For this review, take the finished solid that the model builds, in its own axes (mm). Coordinates: 2 decimals unless noted, no trailing zeros. Order: outer loops, then holes, each group sorted by start corner. A loop starts at its lowest first (then second) coordinate and runs counter-clockwise, first axis right, second up. Notation, with made-up numbers: M 50.5,21.25 L 76.5,21.25 A21 ccw 76.5,29.25 Z; hole C -30,57.5 d10. An arc over 180 degrees is marked long. Use one line per item in the form item = value. Start each with the question number.
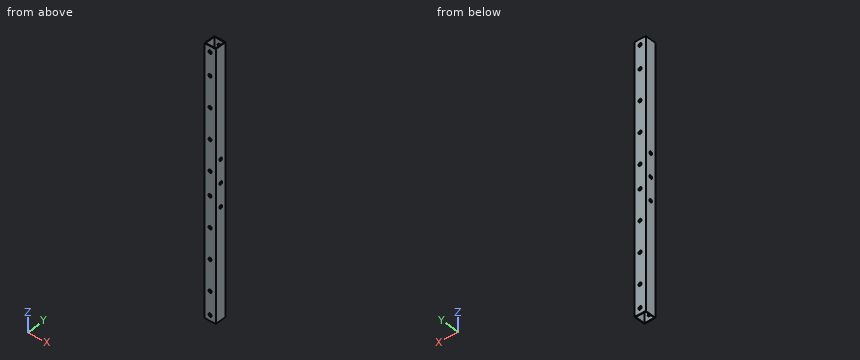
```python
from build123d import *

# Parameters (mm, degrees)
SKETCH_1_W          = 15
SKETCH_1_H          = 15
SKETCH_1_W_2        = 13
SKETCH_1_H_2        = 13
EXTRUDE_1_DEPTH     = 346
SKETCH_3_R          = 2.1
CUT_EXTRUDE_2_DEPTH = 55
SKETCH_4_R          = 2.1
CUT_EXTRUDE_3_DEPTH = 55


with BuildPart() as part:
    # 草图1 → 凸台-拉伸1 (new body)
    with BuildSketch(Plane.XY):
        Rectangle(SKETCH_1_W, SKETCH_1_H)
        Rectangle(SKETCH_1_W_2, SKETCH_1_H_2, mode=Mode.SUBTRACT)
    extrude(amount=EXTRUDE_1_DEPTH)

    # 草图3 → 切除-拉伸2 (cut)
    with BuildSketch(Plane(origin=(0, 7.5, 0), x_dir=(1, 0, 0), z_dir=(0, 1, 0))):
        with Locations(Location((0, -338.5, 0), (0, 0, 270))):
            Circle(SKETCH_3_R)
        with Locations(Location((0, -7.5, 0), (0, 0, 270))):
            Circle(SKETCH_3_R)
        with Locations(Location((0, -37.5, 0), (0, 0, 270))):
            Circle(SKETCH_3_R)
        with Locations(Location((0, -308.5, 0), (0, 0, 270))):
            Circle(SKETCH_3_R)
        with Locations(Location((0, -77.5, 0), (0, 0, 270))):
            Circle(SKETCH_3_R)
        with Locations(Location((0, -117.5, 0), (0, 0, 270))):
            Circle(SKETCH_3_R)
        with Locations(Location((0, -228.5, 0), (0, 0, 270))):
            Circle(SKETCH_3_R)
        with Locations(Location((0, -268.5, 0), (0, 0, 270))):
            Circle(SKETCH_3_R)
        with Locations(Location((0, -157.5, 0), (0, 0, 270))):
            Circle(SKETCH_3_R)
        with Locations(Location((0, -188.5, 0), (0, 0, 270))):
            Circle(SKETCH_3_R)
    extrude(amount=-CUT_EXTRUDE_2_DEPTH, mode=Mode.SUBTRACT)

    # 草图4 → 切除-拉伸3 (cut)
    with BuildSketch(Plane(origin=(7.5, 0, 0), x_dir=(0, 0, -1), z_dir=(1, 0, 0))):
        with Locations((-173, 0)):
            Circle(SKETCH_4_R)
        with Locations((-203, 0)):
            Circle(SKETCH_4_R)
        with Locations((-143, 0)):
            Circle(SKETCH_4_R)
    extrude(amount=-CUT_EXTRUDE_3_DEPTH, mode=Mode.SUBTRACT)


solid = part.part
```
1. To check wall thickness, follow line 1 (Y direction, x = -5.75, z = 119.5); line 2 (X direction, y = -6.9, z = 268.5). State the ranges of each line that lie inside material, in increasing order.
2. Consider section A-A, the plane z = 133.5. Write out the cut boundary in (x, y).
3. For pin 1 Ø6.5 at (x, z) = (0, 117.5) entering from -Y; pin 2 Ø1.5 at (x, y) = (-5, 4.5) entering from +Z, all flat-tipped, find the tip position at first contact; note any pin that passes through.
Answers follow:
q1.line_1 = -7.5 to -6.5, 6.5 to 7.5
q1.line_2 = -7.5 to -2.1, 2.1 to 7.5
q2.outline = M -7.5,-7.5 L 7.5,-7.5 L 7.5,7.5 L -7.5,7.5 Z; hole M -6.5,-6.5 L 6.5,-6.5 L 6.5,6.5 L -6.5,6.5 Z
q3.pin_1 = -7.5
q3.pin_2 = through
